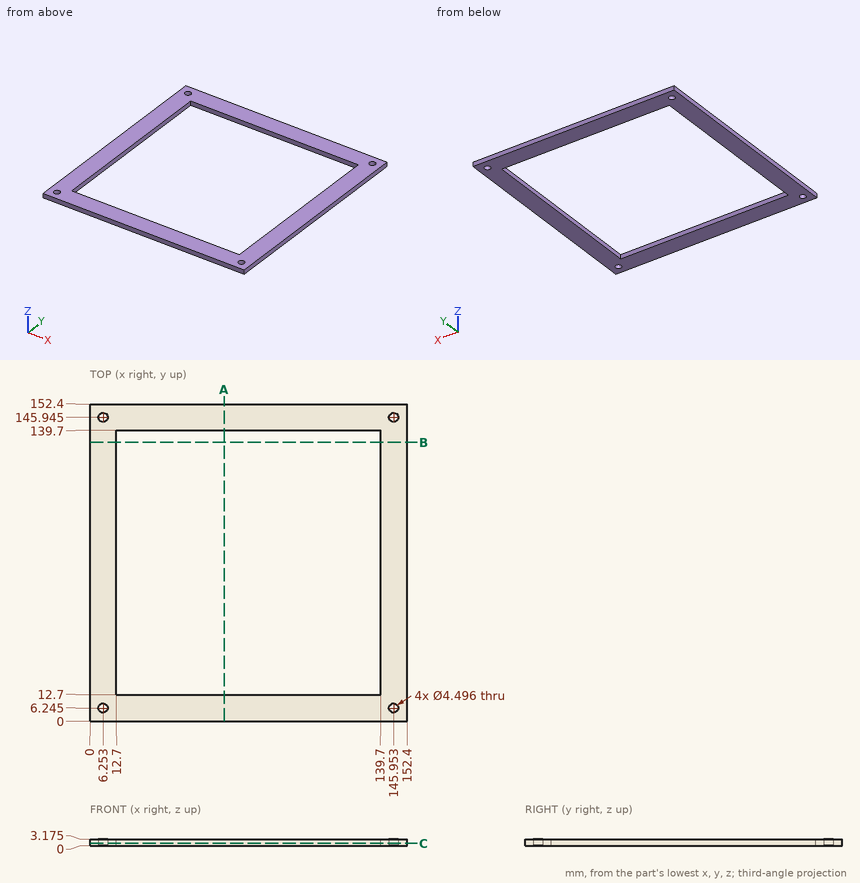
Job drawing, mm, ordinate dimensions from the low corner. One solid piece. Round coordinates to 2 decimals unless told otherwise and drop trailing zeros. Loops run counter-clockwise (first coordinate to the right, second up) from the corner with the lowest first, then second, coordinate; pieces in that order, holes last.
Item 1: Cut at A-A, the plane x = 64.5. Give the cut face in (y, z) (1 decimal).
Item 2: Drill centre lines: line 1 (X direction, y = 97, z = 2.2); line 2 (Y direction, x = 145.5, z = 0.75). Where is each one in solid material? Low to high.
Item 3: Drop a flat-ended pin along its axis: P1, Ø4, axis at x = 6.25, y = 6.25, coming from the -Z side (1 decimal). Give the stop position or say it passes through.
Item 4: Cut at C-C, the plane z = 1.1. Give the cut face in (x, y) (1 decimal).
A:
1. outline: (0, 0) - (12.7, 0) - (12.7, 3.2) - (0, 3.2) - close; (139.7, 0) - (152.4, 0) - (152.4, 3.2) - (139.7, 3.2) - close
2. line 1: x = 0 to 12.7, 139.7 to 152.4
2. line 2: y = 0 to 4.04, 8.45 to 143.74, 148.15 to 152.4
3. P1: passes through
4. outline: (0, 0) - (152.4, 0) - (152.4, 152.4) - (0, 152.4) - close; hole circle Ø4.5 at (6.3, 6.2); hole circle Ø4.5 at (6.3, 145.9); hole (12.7, 12.7) - (139.7, 12.7) - (139.7, 139.7) - (12.7, 139.7) - close; hole circle Ø4.5 at (146, 6.2); hole circle Ø4.5 at (146, 145.9)
